from build123d import *

# Parameters (mm, degrees)
BOSS_EXTRUDE1_DEPTH = 15
CUT_EXTRUDE1_DEPTH  = 5
SKETCH3_R           = 0.75
CUT_EXTRUDE2_DEPTH  = 30
CUT_EXTRUDE3_DEPTH  = 5


with BuildPart() as part:
    # Sketch1 → Boss-Extrude1 (new body)
    with BuildSketch(Plane(origin=(0, 0, 0), x_dir=(1, 0, 0), z_dir=(0, 1, 0))):
        Polygon((0, 0), (210, 0), (180, 30), (30, 30), align=None)
    extrude(amount=BOSS_EXTRUDE1_DEPTH)

    # Sketch2 → Cut-Extrude1 (cut)
    with BuildSketch(Plane(origin=(0, 15, 0), x_dir=(1, 0, 0), z_dir=(0, 1, 0))):
        with BuildLine():
            Line((-5, 22.5), (35, 22.5))
            ThreePointArc((35, 22.5), (42.5, 15), (35, 7.5))
            Line((35, 7.5), (-5, 7.5))
            ThreePointArc((-5, 7.5), (-12.5, 15), (-5, 22.5))
        make_face()
        with BuildLine():
            Line((215, 22.5), (175, 22.5))
            ThreePointArc((175, 22.5), (167.5, 15), (175, 7.5))
            Line((175, 7.5), (215, 7.5))
            ThreePointArc((215, 7.5), (222.5, 15), (215, 22.5))
        make_face()
    extrude(amount=-CUT_EXTRUDE1_DEPTH, mode=Mode.SUBTRACT)

    # Sketch3 → Cut-Extrude2 (cut)
    with BuildSketch(Plane.XY):
        with Locations((105, 7.5)):
            Circle(SKETCH3_R)
        with Locations((52.5, 7.5)):
            Circle(SKETCH3_R)
        with Locations((157.5, 7.5)):
            Circle(SKETCH3_R)
    extrude(amount=-CUT_EXTRUDE2_DEPTH, mode=Mode.SUBTRACT)

    # Sketch4 → Cut-Extrude3 (cut)
    with BuildSketch(Plane(origin=(0, 15, 0), x_dir=(1, 0, 0), z_dir=(0, 1, 0))):
        with BuildLine():
            Line((52.5, 25), (157.5, 25))
            ThreePointArc((157.5, 25), (161.035533906, 23.535533906), (162.5, 20))
            Line((162.5, 20), (162.5, 10))
            ThreePointArc((162.5, 10), (161.035533906, 6.464466094), (157.5, 5))
            Line((157.5, 5), (52.5, 5))
            ThreePointArc((52.5, 5), (48.964466094, 6.464466094), (47.5, 10))
            Line((47.5, 10), (47.5, 20))
            ThreePointArc((47.5, 20), (48.964466094, 23.535533906), (52.5, 25))
        make_face()
    extrude(amount=-CUT_EXTRUDE3_DEPTH, mode=Mode.SUBTRACT)


solid = part.part
Build history of the part. All positions in model axes, mm. A direction names the side the tool comes from. Coordinates: 2 decimals unless noted, no trailing zeros. Order: outer loops, then holes, each group sorted by start corner. A loop starts at its lowest first (then second) coordinate and runs counter-clockwise, first axis right, second up. Notation, with made-up numbers: (-21, 42) -> (15, 42) arc R26 ccw to (15, 57) -> close; hole circle Ø9 at (-13.75, 19). An arc over 180 degrees is marked (long way). One line per item, written item: value.
(1) Slice it at A-A, the plane z = -15. List the corners of the cut face in (x, y).
Checked values:
outline: (15, 0) -> (195, 0) -> (195, 10) -> (167.5, 10) -> (167.5, 15) -> (162.5, 15) -> (162.5, 10) -> (47.5, 10) -> (47.5, 15) -> (42.5, 15) -> (42.5, 10) -> (15, 10) -> close; hole circle Ø1.5 at (52.5, 7.5); hole circle Ø1.5 at (105, 7.5); hole circle Ø1.5 at (157.5, 7.5)
(2) Mould opens along X. For faces 5 (the flat face through (104, 13, -25)), 6 (the flat face through (106, 7, -30)), 7 (the flat face through (15, 6, -15)), 8 (the cylindrical face through (167.5, 12.54, -15.16)) say: pulls with the +X half, pulls with the -X half, needs draft (parallel to the pull), parting line crosses it, or undercut.
Checked values:
face 5: undercut
face 6: needs draft
face 7: pulls with the -X half
face 8: pulls with the +X half
(3) Tool access for faces 1 (the flat face through (104, 0, -15)), 2 (the flat face through (189, 13, -7.5)), 3 (the flat face through (29, 10, -15)), 4 (the cylindrical face through (161, 12.54, -23.57)): list every direction of +Z, -Z, +X, -X, +Y, -Y with a clear straight run to the whole face (end or side of a thin tool).
Checked values:
face 1: +Z, -Z, +X, -X, -Y
face 2: +X, +Y
face 3: -X, +Y
face 4: +Y
(4) Slice it at B-B, the plane y = 13.25. List the corners of the cut face in (x, z).
Checked values:
outline: (0, 0) -> (7.5, -7.5) -> (35, -7.5) arc R7.5 cw to (35, -22.5) -> (22.5, -22.5) -> (30, -30) -> (180, -30) -> (187.5, -22.5) -> (175, -22.5) arc R7.5 cw to (175, -7.5) -> (202.5, -7.5) -> (210, 0) -> close; hole (47.5, -20) arc R5 ccw to (52.5, -25) -> (157.5, -25) arc R5 ccw to (162.5, -20) -> (162.5, -10) arc R5 ccw to (157.5, -5) -> (52.5, -5) arc R5 ccw to (47.5, -10) -> close
(5) Drop flat-ended pins along their axis: pin 1 Ø4 at (x, y) = (194.5, 13) entering from -Z; pin 2 Ø6 at (x, z) = (60.5, -14) entering from +Y; pin 3 Ø5.5 at (y, z) = (13, -15) entering from +X. Give the stop position or say it passes through.
Checked values:
pin 1: z = -7.5
pin 2: y = 10
pin 3: x = 168.02
(6) Slice it at D-D, the plane y = 2.75. List the corners of the cut face in (x, z), plus the area to 3 significant figures.
Checked values:
outline: (0, 0) -> (30, -30) -> (180, -30) -> (210, 0) -> close
area: 5,400 mm2
(7) Probe line 1 (Z direction, x = 95, y = 12.5); line 2 (Y direction, x = 52.5, z = -14.5); line 3 (Y direction, x = 157, z = -10). List the from-to ranges inside material, lowest first. Write a range as [from, to].
Checked values:
line 1: [-30, -25], [-5, 0]
line 2: [0, 6.75], [8.25, 10]
line 3: [0, 6.94], [8.06, 10]
(8) Slice it at C-C, the plane x = 26.5. List the corners of the cut face in (y, z), plus the area to 4 significant figures.
Checked values:
outline: (0, -26.5) -> (15, -26.5) -> (15, -22.5) -> (10, -22.5) -> (10, -7.5) -> (15, -7.5) -> (15, 0) -> (0, 0) -> close
area: 322.5 mm2
